from build123d import *

# Parameters (mm, degrees)
SKETCH1_R           = 1.4
BOSS_EXTRUDE1_DEPTH = 19.4
SKETCH2_W           = 2.8
SKETCH2_H           = 7.8
BOSS_EXTRUDE2_DEPTH = 1.8


with BuildPart() as part:
    # Sketch1 → Boss-Extrude1 (new body)
    with BuildSketch(Plane(origin=(0, 0, 0), x_dir=(1, 0, 0), z_dir=(0, 1, 0))):
        with BuildLine():
            Line((-4, 0), (-4, 4))
            Line((-4, 4), (4, 4))
            Line((4, 4), (4, 0))
            ThreePointArc((4, 0), (0, -4), (-4, 0))
        make_face()
        with Locations(Location((0, 0, 0), (0, 0, 270))):
            Circle(SKETCH1_R, mode=Mode.SUBTRACT)
    extrude(amount=BOSS_EXTRUDE1_DEPTH)

    # Sketch2 → Boss-Extrude2 (add)
    with BuildSketch(Plane(origin=(0, 0, -4), x_dir=(-1, 0, 0), z_dir=(0, 0, -1))):
        with Locations((0, 13.15)):
            Rectangle(SKETCH2_W, SKETCH2_H)
    extrude(amount=BOSS_EXTRUDE2_DEPTH)


solid = part.part
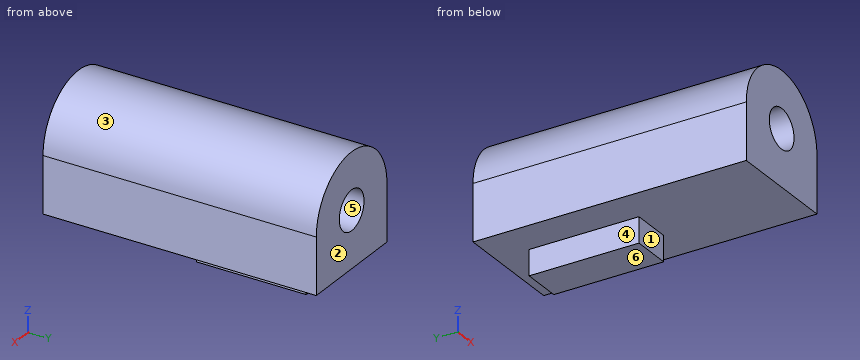
Here's how the part is built. I have some questions about the finished solid (model axes, mm). Face numbers are marked on the shaded views. A direction names the side the tool comes from. Round coordinates to 2 decimals unless told otherwise and drop trailing zeros. Loops run counter-clockwise (first coordinate to the right, second up) from the corner with the lowest first, then second, coordinate; pieces in that order, holes last.
1. Which directions (+Z, -Z, +X, -X, +Y, -Y) give clear straight access to the entire face, cutting with the end or side of a thin tool? Please do the marked faces 1 and 2.
Answer list:
face 1: -Z, +X, -X, -Y
face 2: +Z, -Z, +X, -X, +Y
2. If we section it at C-C on y = 8: Write out the boundary of the cut face in (x, z).
Answer list:
outline: (-4, -4) - (4, -4) - (4, 0) arc R4 ccw to (-4, 0) - close; hole circle Ø2.8 at (0, 0)
3. If we section it at B-B on x = 1: Write out the boundary of the cut face in (y, z), plus the area to 3 significant figures.
Answer list:
outline: (0, -4) - (9.25, -4) - (9.25, -5.8) - (17.05, -5.8) - (17.05, -4) - (19.4, -4) - (19.4, -0.98) - (0, -0.98) - close; (0, 0.98) - (19.4, 0.98) - (19.4, 3.87) - (0, 3.87) - close
area: 129 mm2
4. For P1, Ø2, axis at x = -3, y = 6.5, coming from the -Z side; P2, Ø2.5, axis at x = 0, z = 0, coming from the +Y side; P3, Ø1, axis at y = 3, z = 0.5, coming from the -X side; P4, Ø0.9, axis at x = -0.5, z = -4.5, coming from the -Y side, each with a flat end and sliding along its axis, tell me the tip position at first contact or that it passes through.
Answer list:
P1: stops at z = -4
P2: passes through
P3: stops at x = -4
P4: stops at y = 9.25
5. If we section it at D-D on z = -4.75: Write out the boundary of the cut face in (x, y), plus the area to 3 significant figures.
Answer list:
outline: (-1.4, 9.25) - (1.4, 9.25) - (1.4, 17.05) - (-1.4, 17.05) - close
area: 21.8 mm2
6. If I drill on line 1 along Y through (x, z) = (0, -5); line 2 along X through (y, z) = (1.25, -0.5); line 3 along Z through (x, y) = (0.5, 5), over which ranges is the centre line in solid material (lowest first)?
Answer list:
line 1: y = 9.25 to 17.05
line 2: x = -4 to -1.31, 1.31 to 4
line 3: z = -4 to -1.31, 1.31 to 3.97
7. If we section it at A-A on z = 1: Write out the boundary of the cut face in (x, y), plus the area to 3 significant figures.
Answer list:
outline: (-3.87, 0) - (-0.98, 0) - (-0.98, 19.4) - (-3.87, 19.4) - close; (0.98, 0) - (3.87, 0) - (3.87, 19.4) - (0.98, 19.4) - close
area: 112 mm2
8. We'd pull the mould along Z, two halves only. Please class the marked faces 3, 4, 5 and 6: +Z half, -Z half, draft (parallel to the pull), parting line (faces both ways), or undercut.
Answer list:
face 3: +Z half
face 4: draft
face 5: undercut
face 6: -Z half
